Could you check a few things on this model? Use its own coordinates, in mm. A direction names the side the tool comes from. Give positions to 0.01 mm unless a question says otherwise; leave off trailing zeros. Loops run counter-clockwise (first coordinate to the right, second up) from the corner with the lowest first, then second, coordinate; pieces in that order, holes last. Notation, with made-up numbers: M 78,-3.75 L 105,-3.75 A28 ccw 105,15.25 Z; hole C -29,77.5 d11. An arc over 180 degrees is marked long. Use a Markdown table: item, result. Add a question column.
1) Will these pins go through, and if not, where does the flat tip stop? pin 1 Ø7 at (y, z) = (145, 4) entering from -X (3 decimals); pin 2 Ø1.5 at (y, z) = (102.5, 12.5) entering from -X; pin 3 Ø1 at (y, z) = (43, -0.5) entering from +X.
2) If I drill on line 1 along Z through (x, y) = (-80, 6.5); line 2 along X through (y, z) = (4, -20); line 3 along Y through (x, z) = (22, 0), over which ranges is the centre line in solid material (lowest first)? Write a range as [from, to].
3) Which directions (+Z, -Z, +X, -X, +Y, -Y) give clear straight access to the entire face, cutting with the end or side of a thin tool? Please do faces 1 (the flat face through (0, 115.803, 0)), 2 (the flat face through (-35.711, 151, 0)), 3 (the flat face through (45.115, 151, 0)).
4) We'd pull the mould along X, two halves only. Please class faces 4 (the flat face through (42, 170.383, 0)), 5 (the cylindrical face through (42.619, 4.92, -17.992)), 6 (the flat face through (-45.115, 150, 0)): +X half, -X half, draft (parallel to the pull), parting line (faces both ways), or undercut.
5) Suppose I cut it at A-A on x = -80. List the corners of the cut face in (y, z) for me (3 decimals).
6) Suppose I cut it at C-C on x = 0. List the corners of the cut face in (y, z) for me (3 decimals).
7) Suppose I cut it at D-D on y = 103. List the corners of the cut face in (x, z) for me, and give its area (3 significant figures).
8) Suppose I cut it at B-B on z = 20. List the corners of the cut face in (x, y) for me (3 decimals), and give its area (3 significant figures).
```python
from build123d import *

# Parameters (mm, degrees)
SKETCH1_W                      = 174
SKETCH1_H                      = 50
BOSS_EXTRUDE1_DEPTH            = 10
M6_CLEARANCE_HOLE1_D           = 6.6
M6_CLEARANCE_HOLE1_CSINK_D     = 6.65
M6_CLEARANCE_HOLE1_CSINK_ANGLE = 100
BOSS_EXTRUDE2_DEPTH            = 12
BOSS_EXTRUDE2_DEPTH_BACK       = 12
CUT_EXTRUDE1_REACH             = 215.496
SKETCH7_W                      = 90.229970364
SKETCH7_H                      = 70
SKETCH8_R                      = 15.08125
CUT_EXTRUDE2_DEPTH             = 5.56
SKETCH9_R                      = 11.905
CUT_EXTRUDE3_DEPTH             = 11.1
SKETCH10_W                     = 26.063735182
SKETCH10_H                     = 24
BOSS_EXTRUDE3_DEPTH            = 36.25
CUT_EXTRUDE4_START             = -24.61125
SKETCH11_R                     = 15.08
CUT_EXTRUDE4_DEPTH             = 49.2225
CUT_EXTRUDE5_DEPTH             = 35.71125
CUT_EXTRUDE5_DEPTH_BACK        = 35.71125
SKETCH12_R                     = 11.905
SKETCH13_W                     = 6.477
SKETCH13_H                     = 19.05
CUT_EXTRUDE6_DEPTH             = 0.64
M2_CLEARANCE_HOLE1_D           = 2.6
M2_CLEARANCE_HOLE1_DEPTH       = 2
M2_CLEARANCE_HOLE1_TIP         = 0.781118805
SKETCH16_W                     = 6.477
SKETCH16_H                     = 24
BOSS_EXTRUDE4_DEPTH            = 1.67


with BuildPart() as part:
    # Sketch1 → Boss-Extrude1 (new body)
    with BuildSketch(Plane(origin=(0, 0, 0), x_dir=(1, 0, 0), z_dir=(0, 1, 0))):
        Rectangle(SKETCH1_W, SKETCH1_H)
    extrude(amount=BOSS_EXTRUDE1_DEPTH)

    # M6 Clearance Hole1 (through all)
    with Locations(Plane(origin=(0, 10, 0), x_dir=(1, 0, 0), z_dir=(0, 1, 0))):
        with Locations((-80, 20), (-40, 20), (-80, -20), (-40, -20), (40, 20), (80, 20), (40, -20), (80, -20)):
            CounterSinkHole(M6_CLEARANCE_HOLE1_D / 2, M6_CLEARANCE_HOLE1_CSINK_D / 2, counter_sink_angle=M6_CLEARANCE_HOLE1_CSINK_ANGLE)

    # Sketch6 → Boss-Extrude2 (add, two sides: drawn at the far end of the back side and taken through both)
    with BuildSketch(Plane.XY.offset(-BOSS_EXTRUDE2_DEPTH_BACK)):
        with BuildLine():
            Line((-72, 10), (72, 10))
            Line((72, 10), (39.069577731, 160))
            ThreePointArc((39.069577731, 160), (0, 191.422815383), (-39.069577731, 160))
            Line((-39.069577731, 160), (-72, 10))
        make_face()
    extrude(amount=BOSS_EXTRUDE2_DEPTH + BOSS_EXTRUDE2_DEPTH_BACK)

    # Sketch7 → Cut-Extrude1 (cut, up to next)
    with BuildSketch(Plane.XY.offset(12), mode=Mode.PRIVATE) as cut_extrude1_sk1:
        with Locations((0, 167.46281538)):
            Rectangle(SKETCH7_W, SKETCH7_H)
    cut_extrude1_tool1 = extrude(cut_extrude1_sk1.sketch, amount=-CUT_EXTRUDE1_REACH, mode=Mode.PRIVATE) & part.part
    add(cut_extrude1_tool1.solids().sort_by_distance((0, 167.462815, 12))[0], mode=Mode.SUBTRACT)

    # Sketch8 → Cut-Extrude2 (cut)
    with BuildSketch(Plane(origin=(0, 132.46281538, 0), x_dir=(1, 0, 0), z_dir=(0, 1, 0))):
        Circle(SKETCH8_R)
    extrude(amount=-CUT_EXTRUDE2_DEPTH, mode=Mode.SUBTRACT)

    # Sketch9 → Cut-Extrude3 (cut)
    with BuildSketch(Plane(origin=(0, 126.90281538, 0), x_dir=(1, 0, 0), z_dir=(0, 1, 0))):
        with Locations(Location((0, 0, 0), (0, 0, 270))):
            Circle(SKETCH9_R)
    extrude(amount=-CUT_EXTRUDE3_DEPTH, mode=Mode.SUBTRACT)

    # Sketch10 → Boss-Extrude3 (add)
    with BuildSketch(Plane(origin=(0, 132.46281538, 0), x_dir=(1, 0, 0), z_dir=(0, 1, 0))):
        with Locations((-32.083117591, 0)):
            Rectangle(SKETCH10_W, SKETCH10_H)
        with Locations((32.083117591, 0)):
            Rectangle(SKETCH10_W, SKETCH10_H)
    extrude(amount=BOSS_EXTRUDE3_DEPTH)

    # Sketch11 → Cut-Extrude4 (cut)
    with BuildSketch(Plane(origin=(0, 0, 0), x_dir=(0, 0, -1), z_dir=(1, 0, 0)).offset(CUT_EXTRUDE4_START)):
        with Locations((0, 151.42281538)):
            Circle(SKETCH11_R)
    extrude(amount=CUT_EXTRUDE4_DEPTH, mode=Mode.SUBTRACT)

    # Sketch12 → Cut-Extrude5 (cut, two sides: drawn at the far end of the back side and taken through both)
    with BuildSketch(Plane(origin=(0, 0, 0), x_dir=(0, 0, -1), z_dir=(1, 0, 0)).offset(-CUT_EXTRUDE5_DEPTH_BACK)):
        with Locations(Location((0, 151.42281538, 0), (0, 0, 180))):
            Circle(SKETCH12_R)
    extrude(amount=CUT_EXTRUDE5_DEPTH + CUT_EXTRUDE5_DEPTH_BACK, mode=Mode.SUBTRACT)

    # Sketch13 → Cut-Extrude6 (cut)
    with BuildSketch(Plane(origin=(0, 168.71281538, 0), x_dir=(1, 0, 0), z_dir=(0, 1, 0))):
        with Locations((-41.876485182, 0)):
            Rectangle(SKETCH13_W, SKETCH13_H)
    extrude(amount=-CUT_EXTRUDE6_DEPTH, mode=Mode.SUBTRACT)

    # M2 Clearance Hole1
    with Locations(Plane(origin=(0, 168.07281538, 0), x_dir=(1, 0, 0), z_dir=(0, 1, 0))):
        with Locations((-41.876485182, 5.565), (-41.876485182, -5.565)):
            Hole(M2_CLEARANCE_HOLE1_D / 2, depth=M2_CLEARANCE_HOLE1_DEPTH)
            with Locations((0, 0, -(M2_CLEARANCE_HOLE1_DEPTH + M2_CLEARANCE_HOLE1_TIP / 2))):  # 118° drill point
                Cone(0, M2_CLEARANCE_HOLE1_D / 2, M2_CLEARANCE_HOLE1_TIP, mode=Mode.SUBTRACT)

    # Sketch16 → Boss-Extrude4 (add)
    with BuildSketch(Plane(origin=(0, 168.71281538, 0), x_dir=(1, 0, 0), z_dir=(0, 1, 0))):
        with Locations((41.876485182, 0)):
            Rectangle(SKETCH16_W, SKETCH16_H)
    extrude(amount=BOSS_EXTRUDE4_DEPTH)


solid = part.part
```
Answer block:
| question | item | result |
|---|---|---|
| 1 | pin 1 | stops at x = -45.115 |
| 1 | pin 2 | stops at x = -51.82 |
| 1 | pin 3 | stops at x = 64.87 |
| 2 | line 1 | z = [-25, -23.3], [-16.7, 16.7], [23.3, 25] |
| 2 | line 2 | x = [-87, -83.3], [-76.7, -43.3], [-36.7, 36.7], [43.3, 76.7], [83.3, 87] |
| 2 | line 3 | y = [0, 136.34], [166.5, 168.71] |
| 3 | face 1 | +Y |
| 3 | face 2 | none |
| 3 | face 3 | +Z, -Z, +X, +Y |
| 4 | face 4 | draft |
| 4 | face 5 | undercut |
| 4 | face 6 | -X half |
| 5 | outline | M 0,-25 L 10,-25 L 10,-23.325 L 9.979,-23.3 L 0,-23.3 Z; M 0,-16.7 L 9.979,-16.7 L 10,-16.675 L 10,16.675 L 9.979,16.7 L 0,16.7 Z; M 0,23.3 L 9.979,23.3 L 10,23.325 L 10,25 L 0,25 Z |
| 6 | outline | M 0,-25 L 10,-25 L 10,-12 L 126.903,-12 L 126.903,-11.905 L 115.803,-11.905 L 115.803,11.905 L 126.903,11.905 L 126.903,12 L 10,12 L 10,25 L 0,25 Z |
| 7 | outline | M -51.58,-12 L 51.58,-12 L 51.58,12 L -51.58,12 Z |
| 7 | area | 2,480 mm^2 |
| 8 | outline | M -87,0 L -83.3,0 L -83.3,9.979 L -83.325,10 L -87,10 Z; M -76.7,0 L -43.3,0 L -43.3,9.979 L -43.325,10 L -76.675,10 L -76.7,9.979 Z; M -36.7,0 L 36.7,0 L 36.7,9.979 L 36.675,10 L -36.675,10 L -36.7,9.979 Z; M 43.3,0 L 76.7,0 L 76.7,9.979 L 76.675,10 L 43.325,10 L 43.3,9.979 Z; M 83.3,0 L 87,0 L 87,10 L 83.325,10 L 83.3,9.979 Z |
| 8 | area | 1,480 mm^2 |
